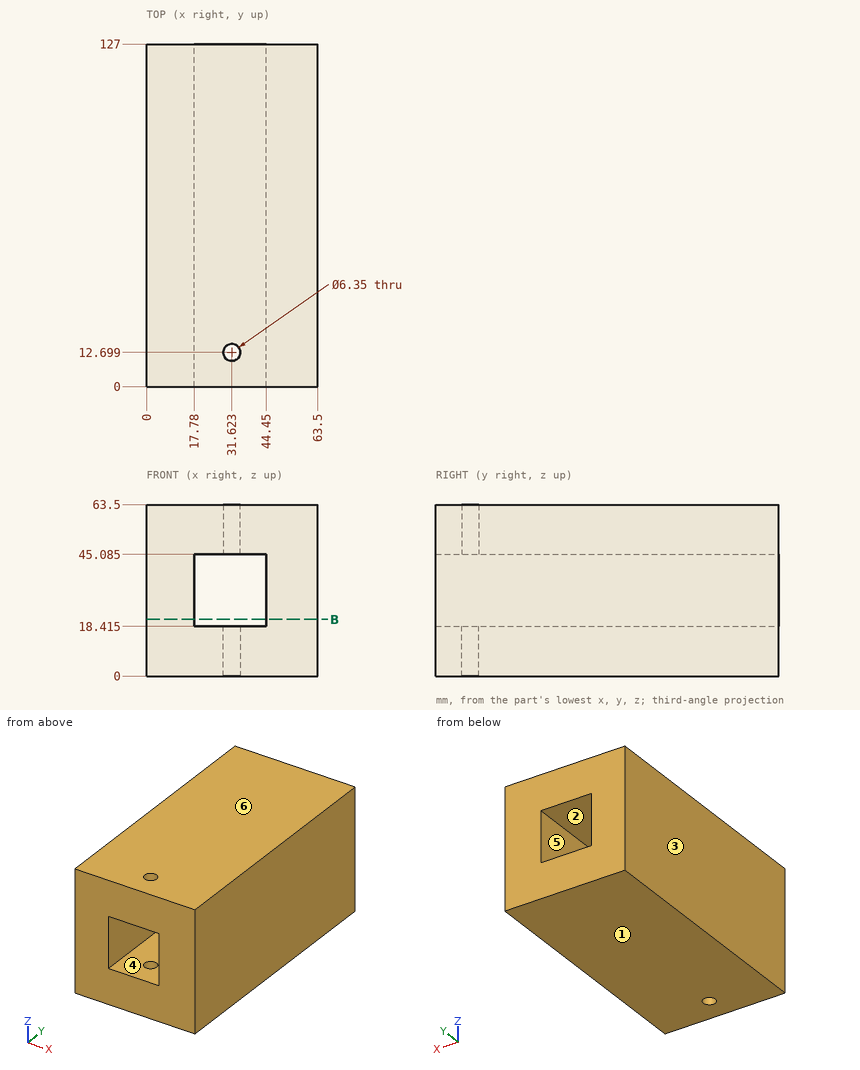
Geometry check sheet. Reference: drawing and pictorial views, mm from the part's lowest x, y, z. A direction names the side the tool comes from. Round coordinates to 2 decimals unless told otherwise and drop trailing zeros. Loops run counter-clockwise (first coordinate to the right, second up) from the corner with the lowest first, then second, coordinate; pieces in that order, holes last. Notation, with made-up numbers: (33, 50.5) - (67, 50.5) arc R12 cw to (67, 68.5) - close; hole circle Ø9 at (74, 25.25). An arc over 180 degrees is marked (long way). Use a Markdown table: item, result. Add a question column.
1. Gauge pin test, flat end, axial feed: pin 1 (4 mm diameter, centred on x = 31.62, y = 12.7, fed in from +Z). Record the tip position at first contact, or that the pin passes through.
2. Section check B-B, the plane z = 21. Record the boundary of the cut face in (x, y).
3. Access from +Z, -Z, +X, -X, +Y, -Y to the whole of each face (thin tool, end or side, straight path). Record for the marked faces 1 and 2.
4. Release check for a two-part mould opening along Z. For the marked faces 3, 4, 5 and 6 record: released by +Z, released by -Z, zero draft, split by the parting line, or undercut.
5. Thickness scan on probe 1 along X at (y, z) = (17, 29.5); probe 2 along Z at (x, y) = (44, 20) (1 decimal). Record the ranges inside material, lowest first. Write a range as [from, to].
Checks:
| question | item | result |
|---|---|---|
| 1 | pin 1 | passes through |
| 2 | outline | (0, 0) - (17.78, 0) - (17.78, 127) - (0, 127) - close; (44.45, 0) - (63.5, 0) - (63.5, 127) - (44.45, 127) - close |
| 3 | face 1 | -Z, +X, -X, +Y, -Y |
| 3 | face 2 | +Y, -Y |
| 4 | face 3 | zero draft |
| 4 | face 4 | undercut |
| 4 | face 5 | undercut |
| 4 | face 6 | released by +Z |
| 5 | probe 1 | x = [0, 17.78], [44.45, 63.5] |
| 5 | probe 2 | z = [0, 18.4], [45.1, 63.5] |
